The model under review builds one solid part; all positions refer to its coordinate system, in mm. Face numbers are marked on the shaded views. A direction names the side the tool comes from. Coordinates: 2 decimals unless noted, no trailing zeros. Loops run counter-clockwise (first coordinate to the right, second up) from the corner with the lowest first, then second, coordinate; pieces in that order, holes last. Notation, with made-up numbers: (59, 62) - (101, 62) arc R23 cw to (101, 85) - close; hole circle Ø7 at (38, -32.75). An arc over 180 degrees is marked (long way). Answer in a Markdown table with one row per item. Add a question column.
(1) We need section C-C on y = 38.1. Write out the cut boundary in (x, z).
(2) For P1, Ø4.5, axis at y = -24.5, z = 23.5, coming from the +X side; P2, Ø4, axis at x = 5.5, y = 7, coming from the +Z side; P3, Ø2, axis at y = 24.5, z = 23.5, coming from the +X side, all flat-tipped, find the tip position at first contact; note any pin that passes through.
(3) We need section D-D on x = 1.25. Write out the cut boundary in (y, z).
(4) We need section A-A on y = -24.5. Write out the cut boundary in (x, z), plus the area to 3 significant figures.
(5) We need section B-B on z = 81.5. Write out the cut boundary in (x, y), plus the area to 3 significant figures.
(6) Machinability: for the marked faces 1 and 2, which of the approach directions +Z, -Z, +X, -X, +Y, -Y give a long, thin tool a straight path to every point of the face, cutting with its end or side? Answer none if there is none.
(7) For line 1 along Z through (x, y) = (-8.5, 24.5); line 2 along Y through (x, z) = (-9.6, 81.5); line 3 along Z through (x, y) = (5.75, -36), list the stretches that pass through material, from the lowest coordinate up.
from build123d import *

# Parameters (mm, degrees)
SKETCH_W     = 15.88
SKETCH_H     = 88.9
SKETCH_R     = 2.775
PAD_DEPTH    = 2.2
SKETCH001_W  = 88.9
SKETCH001_H  = 85
SKETCH001_R  = 1.35
PAD001_DEPTH = 2.2


with BuildPart() as part:
    # Sketch → Pad (new body)
    with BuildSketch(Plane.XY):
        Rectangle(SKETCH_W, SKETCH_H)
        with Locations((-0.0025, 38.1)):
            Circle(SKETCH_R, mode=Mode.SUBTRACT)
        with Locations((-0.0025, -38.1)):
            Circle(SKETCH_R, mode=Mode.SUBTRACT)
    extrude(amount=PAD_DEPTH)

    # Sketch001 (on Face4 of Pad) → Pad001 (join)
    with BuildSketch(Plane(origin=(-7.94, 0, 0), x_dir=(0, -1, 0), z_dir=(-1, 0, 0))):
        with Locations((0, 42.5)):
            Rectangle(SKETCH001_W, SKETCH001_H)
        with Locations((-24.5, 23.5)):
            Circle(SKETCH001_R, mode=Mode.SUBTRACT)
        with Locations((24.5, 23.5)):
            Circle(SKETCH001_R, mode=Mode.SUBTRACT)
        with Locations((24.5, 81.5)):
            Circle(SKETCH001_R, mode=Mode.SUBTRACT)
        with Locations((-24.5, 81.5)):
            Circle(SKETCH001_R, mode=Mode.SUBTRACT)
    extrude(amount=PAD001_DEPTH)


solid = part.part
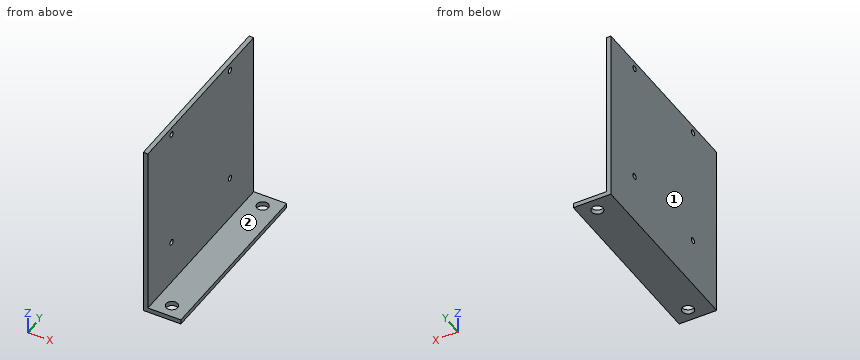
Outcome:
| question | item | result |
|---|---|---|
| 1 | outline | (-10.14, 0) - (-2.78, 0) - (-2.78, 2.2) - (-7.94, 2.2) - (-7.94, 85) - (-10.14, 85) - close; (2.77, 0) - (7.94, 0) - (7.94, 2.2) - (2.77, 2.2) - close |
| 2 | P1 | x = -7.94 |
| 2 | P2 | z = 2.2 |
| 2 | P3 | through |
| 3 | outline | (-44.45, 0) - (-40.58, 0) - (-40.58, 2.2) - (-44.45, 2.2) - close; (-35.62, 0) - (35.62, 0) - (35.62, 2.2) - (-35.62, 2.2) - close; (40.58, 0) - (44.45, 0) - (44.45, 2.2) - (40.58, 2.2) - close |
| 4 | outline | (-10.14, 0) - (7.94, 0) - (7.94, 2.2) - (-7.94, 2.2) - (-7.94, 22.15) - (-10.14, 22.15) - close; (-10.14, 24.85) - (-7.94, 24.85) - (-7.94, 80.15) - (-10.14, 80.15) - close; (-10.14, 82.85) - (-7.94, 82.85) - (-7.94, 85) - (-10.14, 85) - close |
| 4 | area | 210 mm² |
| 5 | outline | (-10.14, -44.45) - (-7.94, -44.45) - (-7.94, -25.85) - (-10.14, -25.85) - close; (-10.14, -23.15) - (-7.94, -23.15) - (-7.94, 23.15) - (-10.14, 23.15) - close; (-10.14, 25.85) - (-7.94, 25.85) - (-7.94, 44.45) - (-10.14, 44.45) - close |
| 5 | area | 184 mm² |
| 6 | face 1 | +Z, -Z, -X, +Y, -Y |
| 6 | face 2 | +Z, +X, +Y, -Y |
| 7 | line 1 | 0 to 22.15, 24.85 to 80.15, 82.85 to 85 |
| 7 | line 2 | -44.45 to -25.85, -23.15 to 23.15, 25.85 to 44.45 |
| 7 | line 3 | 0 to 2.2 |
